Could you check a few things on this model? Use its own coordinates, in mm. Face numbers are marked on the shaded views. A direction names the side the tool comes from. Round coordinates to 2 decimals unless told otherwise and drop trailing zeros. Order: outer loops, then holes, each group sorted by start corner. A loop starts at its lowest first (then second) coordinate and runs counter-clockwise, first axis right, second up. Notation, with made-up numbers: (65.25, 1) -> (71.25, 1) arc R31 cw to (71.25, 34) -> close; hole circle Ø6 at (-18.75, -21). An arc over 180 degrees is marked (long way). Put each result on its own line as item: value. Start each with the question number.
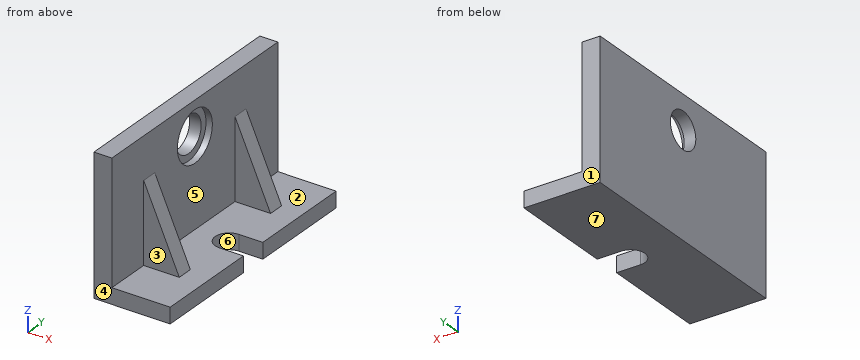
from build123d import *

# Parameters (mm, degrees)
F1_DEPTH  = 76.2
F2_R      = 11.6445519737
F3_DEPTH  = 12.7
F4_R      = 16.0689830222
F4_R_2    = 11.6445519737
F5_DEPTH  = 4.064
F7_DEPTH  = 10.0515203009
F10_DEPTH = 10.16


# Not quite as in the source:
# - a pattern or mirror of a feature is missing from the dataset's text; its kind, count and spacing are read off the source's solid


with BuildPart() as f1:
    # F0 (on Front) → F1 (new body, symmetric)
    with BuildSketch(Plane.XZ):
        Polygon((-46.9024144113, -27.3925848305), (-46.9024144113, 50.0555187464), (-58.332413435, 50.0555187464), (-58.332413435, -37.4431051314), (-9.8534487188, -37.4431051314), (-9.8534487188, -27.3925848305), align=None)
    extrude(amount=F1_DEPTH, both=True)

    # F2 (on face) → F3 (cut, symmetric)
    with BuildSketch(Plane.YZ.offset(-46.9024144113)):
        with Locations((0, 28.3396150917)):
            Circle(F2_R)
    extrude(amount=F3_DEPTH, both=True, mode=Mode.SUBTRACT)

    # F4 (on face) → F5 (cut)
    with BuildSketch(Plane.YZ.offset(-46.9024144113)):
        with Locations((0, 28.3396150917)):
            Circle(F4_R)
        with Locations((0, 28.3396150917)):
            Circle(F4_R_2, mode=Mode.SUBTRACT)
    extrude(amount=-F5_DEPTH, mode=Mode.SUBTRACT)

    # F6 (on face) → F7 (cut, through all)
    with BuildSketch(Plane.XY.offset(-27.3925848305)):
        with BuildLine():
            ThreePointArc((-25.0934487188, -8.89), (-18.807269434, -6.2861792847), (-16.2034487188, 0))
            ThreePointArc((-16.2034487188, 0), (-18.807269434, 6.2861792847), (-25.0934487188, 8.89))
            ThreePointArc((-25.0934487188, 8.89), (-33.9834487188, 0), (-25.0934487188, -8.89))
        make_face()
        with BuildLine():
            ThreePointArc((-25.0934487188, 8.89), (-18.807269434, 6.2861792847), (-16.2034487188, 0))
            ThreePointArc((-16.2034487188, 0), (-18.807269434, -6.2861792847), (-25.0934487188, -8.89))
            Line((-25.0934487188, -8.89), (-9.8534487188, -8.89))
            Line((-9.8534487188, -8.89), (-9.8534487188, 8.89))
            Line((-9.8534487188, 8.89), (-25.0934487188, 8.89))
        make_face()
    extrude(amount=-F7_DEPTH, mode=Mode.SUBTRACT)

    # F9 (on offset) → F10 (join)
    with BuildSketch(Plane.XZ.offset(-46.99)):
        Polygon((-24.2647007108, -27.3925848305), (-46.9024144113, 23.4074151695), (-46.9024144113, -27.3925848305), align=None)
    f10 = extrude(amount=F10_DEPTH)

    # F10_copies: F10 across plane
    add(f10.mirror(Plane(origin=(0, 0, 0), x_dir=(0, 0, -1), z_dir=(0, -1, 0))))


solid = f1.part
1. I need wall thicknesses on L1, parallel to Z at x = -53.5, y = 0; L2, parallel to Z at x = -49, y = 0; L3, parallel to Y at x = -18.5, z = -32.5. Which ranges of each line are inside material? Lowest first, please.
2. For pin 1 Ø10 at (x, y) = (-41, -20) entering from +Z; pin 2 Ø11.5 at (x, z) = (-35.5, -1) entering from -Y; pin 3 Ø4 at (y, z) = (-28, 19.5) entering from +X, each with a flat end and sliding along its axis, tell me the tip position at first contact or that it passes through.
3. Thinking about a two-plate mould opening in Y: for the marked faces 4, 5, 6 and 7, which applies, +Y half, -Y half, draft (parallel to the pull), parting line (faces both ways), or undercut?
4. If we section it at B-B, the plane x = -17.5: Please give me the cut outline in (y, z).
5. Which directions (+Z, -Z, +X, -X, +Y, -Y) give clear straight access to the entire face, cutting with the end or side of a thin tool? Please do the marked faces 1, 2 and 3.
6. If we section it at A-A, the plane y = 0: Please give me the cut outline in (x, z).
7. If we section it at D-D, the plane y = 63: Please give me the cut outline in (x, z), then the cut area to 3 significant figures.
8. If we section it at C-C, the plane z = 35.5: Please give me the cut outline in (x, y), then the cut area to 3 significant figures.
Results below:
1. L1: -37.44 to 16.7, 39.98 to 50.06
1. L2: -37.44 to 12.27, 44.41 to 50.06
1. L3: -76.2 to -8.89, 8.89 to 76.2
2. pin 1: z = -27.39
2. pin 2: y = -46.99
2. pin 3: x = -46.9
3. face 4: -Y half
3. face 5: undercut
3. face 6: undercut
3. face 7: draft
4. outline: (-76.2, -37.44) -> (-8.89, -37.44) -> (-8.89, -27.39) -> (-76.2, -27.39) -> close; (8.89, -37.44) -> (76.2, -37.44) -> (76.2, -27.39) -> (8.89, -27.39) -> close
5. face 1: +Z, -Z, +X, -X, +Y
5. face 2: +Z, +X
5. face 3: +Z, +X, -Y
6. outline: (-58.33, -37.44) -> (-33.98, -37.44) -> (-33.98, -27.39) -> (-46.9, -27.39) -> (-46.9, 12.27) -> (-50.97, 12.27) -> (-50.97, 16.7) -> (-58.33, 16.7) -> close; (-58.33, 39.98) -> (-50.97, 39.98) -> (-50.97, 44.41) -> (-46.9, 44.41) -> (-46.9, 50.06) -> (-58.33, 50.06) -> close
7. outline: (-58.33, -37.44) -> (-9.85, -37.44) -> (-9.85, -27.39) -> (-46.9, -27.39) -> (-46.9, 50.06) -> (-58.33, 50.06) -> close
7. area: 1,370 mm2
8. outline: (-58.33, -76.2) -> (-46.9, -76.2) -> (-46.9, -14.39) -> (-50.97, -14.39) -> (-50.97, -9.18) -> (-58.33, -9.18) -> close; (-58.33, 9.18) -> (-50.97, 9.18) -> (-50.97, 14.39) -> (-46.9, 14.39) -> (-46.9, 76.2) -> (-58.33, 76.2) -> close
8. area: 1,490 mm2
